from build123d import *

# Parameters (mm, degrees)
SKETCH1_R           = 15
SKETCH1_R_2         = 5
BOSS_EXTRUDE1_DEPTH = 10


with BuildPart() as part:
    # Sketch1 → Boss-Extrude1 (new body)
    with BuildSketch(Plane.XY):
        with BuildLine():
            Line((69.33860843, 31.002538298), (33.788342918, 21.476873363))
            ThreePointArc((33.788342918, 21.476873363), (18.788342918, 25.49611125), (7.807580804, 36.476873363))
            Line((7.807580804, 36.476873363), (-18.349364905, 81.782032303))
            ThreePointArc((-18.349364905, 81.782032303), (-33.529523872, 93.43017796), (-52.5, 90.932667397))
            ThreePointArc((-52.5, 90.932667397), (-105, 0), (-52.5, -90.932667397))
            ThreePointArc((-52.5, -90.932667397), (-33.529523872, -93.43017796), (-18.349364905, -81.782032303))
            Line((-18.349364905, -81.782032303), (7.807580804, -36.476873363))
            ThreePointArc((7.807580804, -36.476873363), (18.788342918, -25.49611125), (33.788342918, -21.476873363))
            Line((33.788342918, -21.476873363), (69.33860843, -31.002538298))
            ThreePointArc((69.33860843, -31.002538298), (83.00500475, -25.110060517), (80.427804346, -10.452307591))
            ThreePointArc((80.427804346, -10.452307591), (75.741732949, 0), (80.427804346, 10.452307591))
            ThreePointArc((80.427804346, 10.452307591), (83.00500475, 25.110060517), (69.33860843, 31.002538298))
        make_face()
        Circle(SKETCH1_R, mode=Mode.SUBTRACT)
        with Locations((72.444436972, 19.411428383)):
            Circle(SKETCH1_R_2, mode=Mode.SUBTRACT)
        with Locations(Location((72.444436972, -19.411428383, 0), (0, 0, 180))):
            Circle(SKETCH1_R_2, mode=Mode.SUBTRACT)
        with BuildLine():
            ThreePointArc((-45, 77.942286341), (-90, 0), (-45, -77.942286341))
            ThreePointArc((-45, -77.942286341), (-31.339745962, -74.282032303), (-35, -60.621778265))
            ThreePointArc((-35, -60.621778265), (-70, 0), (-35, 60.621778265))
            ThreePointArc((-35, 60.621778265), (-31.339745962, 74.282032303), (-45, 77.942286341))
        make_face(mode=Mode.SUBTRACT)
    extrude(amount=BOSS_EXTRUDE1_DEPTH)


solid = part.part
Geometry check sheet. Reference: the model listing, model coordinates, mm. A direction names the side the tool comes from. Round coordinates to 2 decimals unless told otherwise and drop trailing zeros. Loops run counter-clockwise (first coordinate to the right, second up) from the corner with the lowest first, then second, coordinate; pieces in that order, holes last.
Item 1: Access from +Z, -Z, +X, -X, +Y, -Y to the whole of each face (thin tool, end or side, straight path). Record for faces 5 (the flat face through (51.812, 26.306, 4.93)), 6 (the cylindrical face through (18.598, -25.607, 4.93)), 7 (the cylindrical face through (-89.99, 1.32, 4.93)).
Item 2: Cross-section at B-B on x = 0. Record the boundary of the cut face in (y, z).
Item 3: Cross-section at D-D on x = -65.5. Record the boundary of the cut face in (y, z).
Item 4: Gauge pin test, flat ends, axial feed: pin 1 (2 mm diameter, centred on x = 62, z = 3.5, fed in from -Y); pin 2 (5 mm diameter, centred on x = -55, y = 67, fed in from +Z); pin 3 (1 mm diameter, centred on y = -11, z = 5, fed in from -X); pin 4 (1.5 mm diameter, centred on y = 5, z = 4, fed in from -X). Record the tip position at first contact, or that the pin passes through.
Item 5: Thickness scan on line 1 (Y direction, x = 72, z = 2.5); line 2 (Y direction, x = 71, z = 4.25); line 3 (X direction, y = 6.5, z = 9.25). Record the ranges inside material, lowest first.
Item 6: Mould release check, pull along X, two halves, no side actions. Record for faces 1 (the flat face through (-5.454, -59.447, 4.93)), 2 (the cylindrical face through (-104.99, 1.54, 4.93)), 3 (the flat face through (51.31, -26.17, 4.93)), 4 (the cylindrical face through (77.214, 20.913, 4.93)): pulls with the +X half, pulls with the -X half, needs draft (parallel to the pull), parting line crosses it, or undercut.
Item 7: Cross-section at A-A on y = 0. Record the boundary of the cut face in (x, z), then the cut area to 3 significant figures.
Item 8: Cross-section at C-C on z = 6. Record the boundary of the cut face in (x, y), then the cut area to 3 significant figures.
Answer sheet:
1. face 5: +Z, -Z, +Y
1. face 6: +Z, -Z, -Y
1. face 7: +Z, -Z
2. outline: (-50, 0) - (-15, 0) - (-15, 10) - (-50, 10) - close; (15, 0) - (50, 0) - (50, 10) - (15, 10) - close
3. outline: (-82.07, 0) - (-61.72, 0) - (-61.72, 10) - (-82.07, 10) - close; (-24.69, 0) - (24.69, 0) - (24.69, 10) - (-24.69, 10) - close; (61.72, 0) - (82.07, 0) - (82.07, 10) - (61.72, 10) - close
4. pin 1: stops at y = -29.3
4. pin 2: passes through
4. pin 3: stops at x = -104.47
4. pin 4: stops at x = -104.91
5. line 1: y = -31.4 to -24.39, -14.43 to 14.43, 24.39 to 31.4
5. line 2: y = -31.32 to -24.2, -14.62 to 14.62, 24.2 to 31.32
5. line 3: x = -104.8 to -89.76, -69.7 to -13.52, 13.52 to 77.34
6. face 1: pulls with the +X half
6. face 2: pulls with the -X half
6. face 3: undercut
6. face 4: undercut
7. outline: (-105, 0) - (-90, 0) - (-90, 10) - (-105, 10) - close; (-70, 0) - (-15, 0) - (-15, 10) - (-70, 10) - close; (15, 0) - (75.74, 0) - (75.74, 10) - (15, 10) - close
7. area: 1,310 mm2
8. outline: (-52.5, -90.93) arc R25 ccw to (-18.35, -81.78) - (7.81, -36.48) arc R30 cw to (33.79, -21.48) - (69.34, -31) arc R12 ccw to (80.43, -10.45) arc R14 cw to (80.43, 10.45) arc R12 ccw to (69.34, 31) - (33.79, 21.48) arc R30 cw to (7.81, 36.48) - (-18.35, 81.78) arc R25 ccw to (-52.5, 90.93) arc R105 ccw to start; hole (-45, -77.94) arc R10 ccw to (-35, -60.62) arc R70 cw to (-35, 60.62) arc R10 ccw to (-45, 77.94) arc R90 ccw to start; hole circle Ø30 at (0, 0); hole circle Ø10 at (72.44, -19.41); hole circle Ø10 at (72.44, 19.41)
8. area: 15,500 mm2
